from build123d import *

# Parameters (mm, degrees)
CUT_EXTRUDE1_DEPTH  = 7
SKETCH3_R           = 5
BOSS_EXTRUDE1_DEPTH = 1
SKETCH4_R           = 6.5
BOSS_EXTRUDE2_DEPTH = 5


with BuildPart() as part:
    # Sketch1 → Revolve1 (revolve)
    with BuildSketch(Plane.XY):
        with BuildLine():
            Line((-8, 0), (0, 0))
            Line((0, 0), (0, 41))
            Line((0, 41), (-4, 41))
            Line((-4, 41), (-4, 26))
            Line((-4, 26), (-6, 26))
            Line((-6, 26), (-6, 19))
            Line((-6, 19), (-8, 19))
            ThreePointArc((-8, 19), (-11, 9.5), (-8, 0))
        make_face()
    revolve(axis=Axis((0, 0, 0), (0, 1, 0)))

    # Sketch2 → Cut-Extrude1 (cut)
    with BuildSketch(Plane(origin=(0, 26, 0), x_dir=(1, 0, 0), z_dir=(0, 1, 0))):
        with BuildLine():
            Line((-3.713074887, 4.713074887), (3.713074887, 4.713074887))
            ThreePointArc((3.713074887, 4.713074887), (0, 6), (-3.713074887, 4.713074887))
        make_face()
        with BuildLine():
            Line((4.713074887, 3.713074887), (4.713074887, -3.713074887))
            ThreePointArc((4.713074887, -3.713074887), (6, 0), (4.713074887, 3.713074887))
        make_face()
        with BuildLine():
            Line((3.713074887, -4.713074887), (-3.713074887, -4.713074887))
            ThreePointArc((-3.713074887, -4.713074887), (0, -6), (3.713074887, -4.713074887))
        make_face()
        with BuildLine():
            Line((-4.713074887, -3.713074887), (-4.713074887, 3.713074887))
            ThreePointArc((-4.713074887, 3.713074887), (-6, 0), (-4.713074887, -3.713074887))
        make_face()
    extrude(amount=-CUT_EXTRUDE1_DEPTH, mode=Mode.SUBTRACT)

    # Sketch3 → Boss-Extrude1 (add)
    with BuildSketch(Plane.XZ):
        Circle(SKETCH3_R)
    extrude(amount=BOSS_EXTRUDE1_DEPTH)

    # Sketch4 → Boss-Extrude2 (add)
    with BuildSketch(Plane(origin=(0, 40, 0), x_dir=(1, 0, 0), z_dir=(0, 1, 0))):
        Circle(SKETCH4_R)
    extrude(amount=-BOSS_EXTRUDE2_DEPTH)


solid = part.part
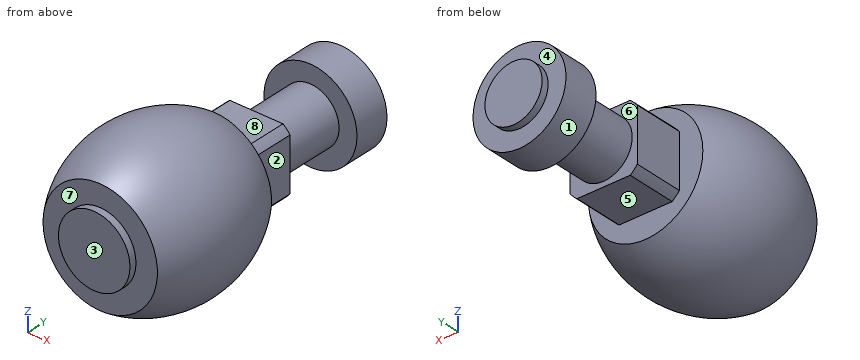
Part model, mm, in its own coordinate system. Face numbers are marked on the shaded views. A direction names the side the tool comes from. Coordinates: 2 decimals unless noted, no trailing zeros. Loops run counter-clockwise (first coordinate to the right, second up) from the corner with the lowest first, then second, coordinate; pieces in that order, holes last. Notation, with made-up numbers: M 19.25,40.25 L 32.25,40.25 A36 ccw 32.25,77.25 Z; hole C -9.75,-34.75 d4. An arc over 180 degrees is marked long. Use a Markdown table: item, result. Add a question column.
Q1. Mould opens along Y. For the marked faces 1, 2, 3 and 4 say: +Y half, -Y half, draft (parallel to the pull), parting line (faces both ways), or undercut.
Q2. Cut at A-A (y = 30.5). Write the cut outline in (x, z).
Q3. Cut at B-B (y = 36.5). Write the cut outline in (x, z).
Q4. Probe L1, parallel to Y at x = 3, z = -5; L2, parallel to Y at x = 4, z = -4; L3, parallel to X at y = 25, z = -2. List the from-to ranges inside material, lowest first.
Q5. Pin check, flat tips, straight feed: P1, Ø4, axis at x = 3, z = -7, coming from the +Y side; P2, Ø5, axis at y = 23.5, z = -6.5, coming from the +X side; P3, Ø4, axis at x = -4.5, y = 5, coming from the -Z side. Stop position of each tip, or through.
Q6. Which spindle directions (+Z, -Z, +X, -X, +Y, -Y) get a long thin tool onto all of the face, cutting with end or side? Do the marked faces 5, 6, 7 and 8. Say none if no direction does.
Worked out:
| question | item | result |
|---|---|---|
| 1 | face 1 | draft |
| 1 | face 2 | undercut |
| 1 | face 3 | -Y half |
| 1 | face 4 | +Y half |
| 2 | outline | C 0,0 d8 |
| 3 | outline | C 0,0 d13 |
| 4 | L1 | y = 0 to 19, 35 to 40 |
| 4 | L2 | y = 0 to 26, 35 to 40 |
| 4 | L3 | x = -4.71 to 4.71 |
| 5 | P1 | stops at y = 40 |
| 5 | P2 | stops at x = 4.47 |
| 5 | P3 | stops at z = -10.27 |
| 6 | face 5 | -Z, +X, -X |
| 6 | face 6 | none |
| 6 | face 7 | -Y |
| 6 | face 8 | +Z, +X, -X |
